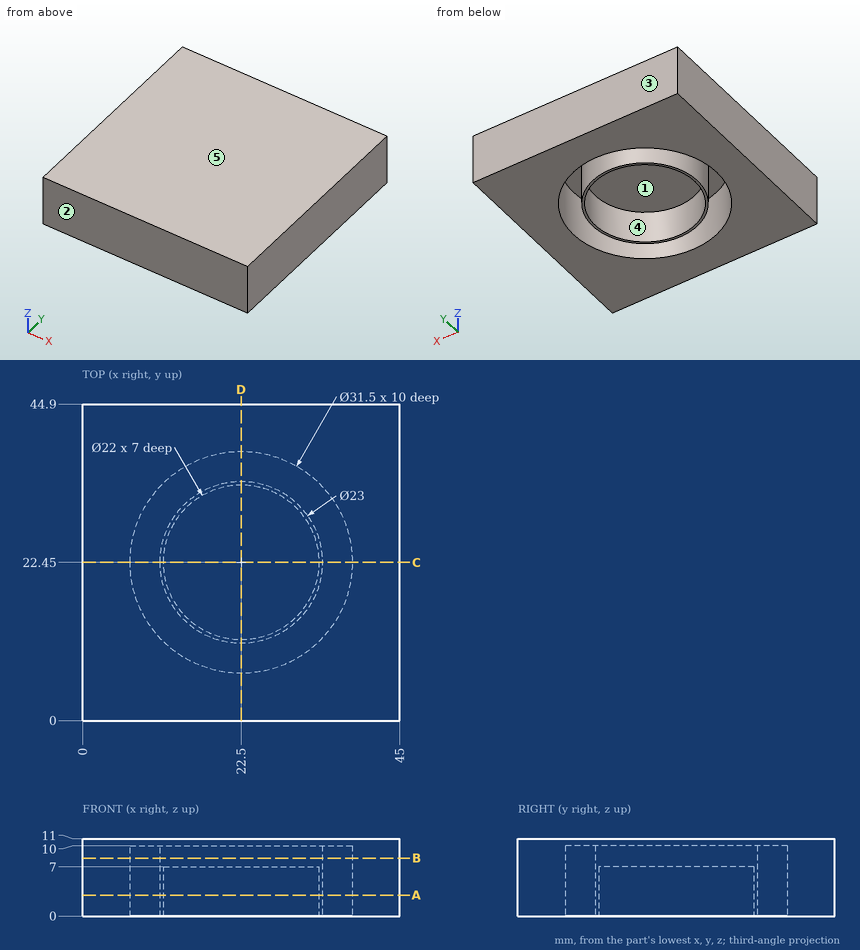
Verification items for this drawing (mm, ordinates from the low corner). A direction names the side the tool comes from. Give positions to 0.01 mm unless a question says otherwise; leave off trailing zeros. Order: outer loops, then holes, each group sorted by start corner. A loop starts at its lowest first (then second) coordinate and runs counter-clockwise, first axis right, second up.
1) Material ranges on probe 1 along Y at (x, z) = (22.5, 1); probe 2 along Y at (x, z) = (15, 6.5); probe 3 along X at (y, z) = (23, 1), recorded low to high.
Results are:
probe 1: y = 0 to 6.7, 10.95 to 11.45, 33.45 to 33.95, 38.2 to 44.9
probe 2: y = 0 to 8.6, 13.73 to 14.4, 30.5 to 31.17, 36.3 to 44.9
probe 3: x = 0 to 6.76, 11.01 to 11.51, 33.49 to 33.99, 38.24 to 45
2) Cross-section at B-B (z = 8.25). Record the boundary of the cut face in (x, y), then the cut area to 3 significant figures.
Results are:
outline: (0, 0) - (45, 0) - (45, 44.9) - (0, 44.9) - close; circle Ø23 at (22.5, 22.45); hole circle Ø31.5 at (22.5, 22.45)
area: 1,660 mm2
3) Cross-section at C-C (y = 22.45). Record the boundary of the cut face in (x, z), then the cut area to 3 significant figures.
Results are:
outline: (0, 0) - (6.75, 0) - (6.75, 10) - (11, 10) - (11, 0) - (11.5, 0) - (11.5, 7) - (33.5, 7) - (33.5, 0) - (34, 0) - (34, 10) - (38.25, 10) - (38.25, 0) - (45, 0) - (45, 11) - (0, 11) - close
area: 256 mm2
4) Cross-section at A-A (z = 3). Record the boundary of the cut face in (x, y).
Results are:
outline: (0, 0) - (45, 0) - (45, 44.9) - (0, 44.9) - close; circle Ø23 at (22.5, 22.45); hole circle Ø31.5 at (22.5, 22.45); hole circle Ø22 at (22.5, 22.45)
5) Draft check along Y on the marked faces 3, 4 and 5. Enter one of: released by +Y, released by -Y, zero draft, split by the parting line, or undercut.
Results are:
face 3: released by +Y
face 4: undercut
face 5: zero draft
6) Cross-section at D-D (x = 22.5). Record the boundary of the cut face in (y, z).
Results are:
outline: (0, 0) - (6.7, 0) - (6.7, 10) - (10.95, 10) - (10.95, 0) - (11.45, 0) - (11.45, 7) - (33.45, 7) - (33.45, 0) - (33.95, 0) - (33.95, 10) - (38.2, 10) - (38.2, 0) - (44.9, 0) - (44.9, 11) - (0, 11) - close
7) Gauge pin test, flat end, axial feed: pin 1 (2 mm diameter, centred on x = 18, y = 20, fed in from -Z). Record the tip position at first contact, or that the pin passes through.
Results are:
pin 1: stops at z = 7
8) Tool access check on the marked faces 1 and 2. Record the directions out of +Z, -Z, +X, -X, +Y, -Y that give a thin tool (end or side, any length) a straight path to the whole face; none if there is none.
Results are:
face 1: -Z
face 2: +Z, -Z, +X, -X, -Y
